For this review, take the finished solid that the model builds, in its own axes (mm). A direction names the side the tool comes from. Coordinates: 2 decimals unless noted, no trailing zeros. Write each loop counter-clockwise with the first axis right and the second up, starting at its lowest first coordinate (ties: lowest second). Pieces come first, ordered by that corner, then holes. Notation, with made-up numbers: (70, 48.25) - (91, 48.25) arc R19 cw to (91, 56.25) - close; hole circle Ø11 at (-9, 65.5). An arc over 180 degrees is marked (long way). Write each question's results on one line, items separated by ' | '.
from build123d import *

# Parameters (mm, degrees)
SKETCH1_R           = 8
BOSS_EXTRUDE1_DEPTH = 172
SKETCH2_R           = 2.5
CUT_EXTRUDE1_DEPTH  = 15
CHAMFER1_SIZE       = 0.5


with BuildPart() as part:
    # Sketch1 → Boss-Extrude1 (new body)
    with BuildSketch(Plane(origin=(0, 0, 0), x_dir=(1, 0, 0), z_dir=(0, 1, 0))):
        Circle(SKETCH1_R)
    extrude(amount=BOSS_EXTRUDE1_DEPTH)

    # Sketch2 → Cut-Extrude1 (cut)
    with BuildSketch(Plane.XZ):
        Circle(SKETCH2_R)
    cut_extrude1 = extrude(amount=-CUT_EXTRUDE1_DEPTH, mode=Mode.SUBTRACT)

    # Mirror1: Cut-Extrude1 across plane
    add(cut_extrude1.mirror(Plane.ZX.offset(86)), mode=Mode.SUBTRACT)

    # Chamfer1
    chamfer1_edges = [part.edges().sort_by_distance(p)[0] for p in [
        (-2.5, 0, 0),
        (-2.5, 172, 0),
    ]]
    chamfer(chamfer1_edges, length=CHAMFER1_SIZE)


solid = part.part
Q1. For faces 4 (the face through (-0.54, 164.35, -2.44)), 5 (the face through (0, 15, 0)), 6 (the face through (3.4, 172, -0.1)), list the 3-axis set-ups (+Z, -Z, +X, -X, +Y, -Y) from which the entire face can be reached by the end or side of a thin tool; tool diameter is ignored.
Results found:
face 4: +Y | face 5: -Y | face 6: +Z, -Z, +X, -X, +Y
Q2. Take a section at B-B on z = 0. State the section outline as (x, y) points.
Results found:
outline: (-8, 0) - (-3, 0) - (-2.5, 0.5) - (-2.5, 15) - (2.5, 15) - (2.5, 0.5) - (3, 0) - (8, 0) - (8, 172) - (3, 172) - (2.5, 171.5) - (2.5, 157) - (-2.5, 157) - (-2.5, 171.5) - (-3, 172) - (-8, 172) - close
Q3. Wall thickness on line 1 along Z through (x, y) = (0, 167.75); line 2 along Z through (x, y) = (-0.25, 58); line 3 along X through (y, z) = (136, -5.5): over which ranges is each line inside the solid? List them lowest first. Write a range as from..to.
Results found:
line 1: -8..-2.5, 2.5..8 | line 2: -8..8 | line 3: -5.81..5.81
Q4. Take a section at A-A on x = 0. State the section outline as (y, z) points.
Results found:
outline: (0, -8) - (172, -8) - (172, -3) - (171.5, -2.5) - (157, -2.5) - (157, 2.5) - (171.5, 2.5) - (172, 3) - (172, 8) - (0, 8) - (0, 3) - (0.5, 2.5) - (15, 2.5) - (15, -2.5) - (0.5, -2.5) - (0, -3) - close
Q5. For pin 1 (3 mm diameter, centred on x = 0, z = 0, fed in from -Y); pin 2 (3 mm diameter, centred on x = 6, y = 105.5, fed in from -Z); pin 3 (5 mm diameter, centred on x = -3.5, y = 130.5, fed in from -Z), all flat-tipped, find the tip position at first contact; note any pin that passes through.
Results found:
pin 1: y = 15 | pin 2: z = -6.61 | pin 3: z = -7.94
Q6. Take a section at C-C on y = 27. State the section outline as (x, z) points.
Results found:
outline: circle Ø16 at (0, 0)
Q7. Mouldability with a two-part tool opening along Z and no side actions: class faces 1 (the face through (-0.54, 7.65, -2.44)), 2 (the face through (-1.73, 84.8, 7.81)), 3 (the face through (3.4, 0, -0.1)) as pulls with the +Z half, pulls with the -Z half, needs draft (parallel to the pull), parting line crosses it, or undercut.
Results found:
face 1: undercut | face 2: parting line crosses it | face 3: needs draft
